from build123d import *

# Parameters (mm, degrees)
F0_R     = 3.429
F1_DEPTH = 4.7752
F3_DEPTH = 4.7762
F4_R     = 0.889
F5_DEPTH = 7.3416
F6_R     = 1.2192
F6_R_2   = 0.889
F7_DEPTH = 2.5908
F8_R     = 0.8001
F9_DEPTH = 4.7752
F10_R    = 4.7752


with BuildPart() as f1:
    # F0 (on Front) → F1 (new body)
    with BuildSketch(Plane.XZ):
        Polygon((0, 9.525), (0, 0), (11.9126, 0), (11.9126, 7.3406), (8.3058, 7.3406), (8.3058, 9.525), align=None)
        with Locations((4.7752, 4.7752)):
            Circle(F0_R, mode=Mode.SUBTRACT)
    extrude(amount=F1_DEPTH)

    # F2 (on face) → F3 (cut, through all)
    with BuildSketch(Plane.XZ.offset(4.7752)):
        with BuildLine():
            Line((11.9126, 5.1816), (8.1800318666, 5.1816))
            ThreePointArc((8.1800318666, 5.1816), (8.1981526341, 4.9787589955), (8.2042, 4.7752))
            ThreePointArc((8.2042, 4.7752), (8.1981526341, 4.5716410045), (8.1800318666, 4.3688))
            Line((8.1800318666, 4.3688), (11.9126, 4.3688))
            Line((11.9126, 4.3688), (11.9126, 5.1816))
        make_face()
    extrude(amount=-F3_DEPTH, mode=Mode.SUBTRACT)

    # F4 (on face) → F5 (cut, through all)
    with BuildSketch(Plane.XY.offset(7.3406)):
        with Locations((10.1854, -2.3876)):
            Circle(F4_R)
    extrude(amount=-F5_DEPTH, mode=Mode.SUBTRACT)

    # F6 (on face) → F7 (cut)
    with BuildSketch(Plane.XY.offset(7.3406)):
        with Locations((10.1854, -2.3876)):
            Circle(F6_R)
        with Locations((10.1854, -2.3876)):
            Circle(F6_R_2, mode=Mode.SUBTRACT)
    extrude(amount=-F7_DEPTH, mode=Mode.SUBTRACT)

    # F8 (on face) → F9 (cut)
    with BuildSketch(Plane(origin=(0, 0, 0), x_dir=(0, -1, 0), z_dir=(-1, 0, 0))):
        with Locations((2.3876, 8.0518)):
            Circle(F8_R)
    extrude(amount=-F9_DEPTH, mode=Mode.SUBTRACT)

    # F10
    f10_edges = [f1.edges().sort_by_distance(p)[0] for p in [
        (0, -2.3876, 0),
    ]]
    fillet(f10_edges, radius=F10_R)


solid = f1.part
Could you check a few things on this model? Use its own coordinates, in mm. A direction names the side the tool comes from. Coordinates: 2 decimals unless noted, no trailing zeros. Loops run counter-clockwise (first coordinate to the right, second up) from the corner with the lowest first, then second, coordinate; pieces in that order, holes last.
1. We'd pull the mould along Y, two halves only. Please class faces 6 (the face through (1.4, -2.4, 1.4)), 7 (the face through (9, -4.775, 4)), 8 (the face through (11.033, -2.121, 2.215)): released by +Y, released by -Y, zero draft, split by the parting line, or undercut.
2. Imagine slicing it at A-A (x = 8.5). Please give me the cut outline in (y, z).
3. For faces 1 (the face through (9, -2, 4.369)), 2 (the face through (11.913, -2, 2)), 3 (the face through (8.306, -2, 8)), 4 (the face through (1.824, -2.283, 8.845)), 5 (the face through (11.348, -2.021, 6.276)), which set-ups out of +Z, -Z, +X, -X, +Y, -Y let a thin tool reach every point of the face, with its end or its side?
4. Imagine slicing it at D-D (x = 10). Please give me the cut outline in (y, z).
5. Imagine slicing it at B-B (z = 5.75). Please give me the cut outline in (x, y), and give its area (3 significant figures).
6. Imagine slicing it at C-C (y = -2.8). Please give me the cut outline in (x, z) (3 decimals).
7. I need wall thicknesses on L1, parallel to Z at x = 11.5, y = -4.45; L2, parallel to X at y = -1.65, z = 6.25; L3, parallel to X at y = -0.3, z = 5.25. Which ranges of each line are inside material? Lowest first, please.
8. For P1, Ø1.1, axis at x = 9.5, y = -2, coming from the +Z side, with a flat end and sliding along its axis, tell me the tip position at first contact or that it passes through.
Computed values:
1. face 6: zero draft
1. face 7: released by -Y
1. face 8: undercut
2. outline: (-4.78, 0) - (0, 0) - (0, 4.37) - (-4.78, 4.37) - close; (-4.78, 5.18) - (0, 5.18) - (0, 7.34) - (-4.78, 7.34) - close
3. face 1: +X, +Y, -Y
3. face 2: +Z, -Z, +X, +Y, -Y
3. face 3: +Z, +X, +Y, -Y
3. face 4: -X
3. face 5: +Z
4. outline: (-4.78, 0) - (-3.26, 0) - (-3.26, 4.37) - (-4.78, 4.37) - close; (-4.78, 5.18) - (-3.59, 5.18) - (-3.59, 7.34) - (-4.78, 7.34) - close; (-1.52, 0) - (0, 0) - (0, 4.37) - (-1.52, 4.37) - close; (-1.18, 5.18) - (0, 5.18) - (0, 7.34) - (-1.18, 7.34) - close
5. outline: (0, -4.78) - (1.49, -4.78) - (1.49, 0) - (0, 0) - close; (8.06, -4.78) - (11.91, -4.78) - (11.91, 0) - (8.06, 0) - close; hole circle Ø2.44 at (10.19, -2.39)
5. area: 20.8 mm2
6. outline: (0, 4.775) arc R4.775 ccw to (4.775, 0) - (9.398, 0) - (9.398, 4.369) - (8.18, 4.369) arc R3.429 cw (long way) to (2.529, 7.366) - (0, 7.366) - close; (0, 8.737) - (4.775, 8.737) - (4.775, 8.204) arc R3.429 cw to (8.18, 5.182) - (9.038, 5.182) - (9.038, 7.341) - (8.306, 7.341) - (8.306, 9.525) - (0, 9.525) - close; (10.973, 0) - (11.913, 0) - (11.913, 4.369) - (10.973, 4.369) - close; (11.333, 5.182) - (11.913, 5.182) - (11.913, 7.341) - (11.333, 7.341) - close
7. L1: z = 0 to 4.37, 5.18 to 7.34
7. L2: x = 0 to 1.68, 7.87 to 9.21, 11.16 to 11.91
7. L3: x = 0 to 1.38, 8.17 to 11.91
8. P1: stops at z = 7.34
